Autodesk Inventor part; units mm, degrees
ref_plane "IP1_XY" through (0, 0, 0) normal (1, 0, 0) x (0, 0, -1)
ref_plane "IP1_YZ" through (0, 0, 0) normal (0, 0, -1) x (0, 1, 0)
ref_plane "IP1_ZX" through (0, 0, 0) normal (0, 1, 0) x (1, 0, 0)
sketch "Skizze_5" plane through (0, 0, 0) normal (0, 0, 1) x (1, 0, 0)
  line L0 (8, 0) -> (0, 0)
  line L1 (0, 0) -> (0, 3.75)
  line L2 (0, 3.75) -> (0.45, 3.75)
  line L3 (0.45, 3.75) -> (2.2, 2)
  line L4 (2.2, 2) -> (7.5705, 2)
  line L5 (7.5705, 2) -> (8, 1.5705)
  line L6 (8, 1.5705) -> (8, 0)
  line L7 (8, 0) -> (0, 0)
revolve "Revolution1" add sketch "Skizze_5" angle 360 about axis through (8, 0, 0) along (1, 0, 0)
thread "Thread1"
sketch "Sketch_1" plane through (0, 0, 0) normal (0, 0, 1) x (1, 0, 0)
  line L0 (1.66, 0) -> (0, 0)
  line L1 (0, 0) -> (0, 1.975)
  line L2 (0, 1.975) -> (1.66, 1.975)
  line L3 (1.66, 1.975) -> (1.66, 0)
  line L4 (1.66, 0) -> (0, 0)
revolve "Revolution2" cut sketch "Sketch_1" angle 360 about axis through (1.66, 0, 0) along (1, 0, 0)
sketch "Sketch_2" plane through (0, 0, 0) normal (0, 0, 1) x (1, 0, 0)
  line L0 (2.8003, 0) -> (1.66, 0)
  line L1 (1.66, 0) -> (1.66, 1.975)
  line L2 (1.66, 1.975) -> (2.8003, 0)
  line L3 (2.8003, 0) -> (1.66, 0)
revolve "Revolution3" cut sketch "Sketch_2" angle 360 about axis through (2.8003, 0, 0) along (1, 0, 0)
sketch "Sketch_3" plane through (0, 0, 0) normal (1, 0, 0) x (0, 1, 0)
  circle A0 centre (0, 0) radius 2.37
  arc A1 (-0.5027, 1.6394) -> (-1.1684, 1.2551) centre (-0.79, 1.3683) ccw
  arc A2 (-1.6711, 0.3843) -> (-1.1684, 1.2551) centre (-1.8307, 1.0569) ccw
  arc A3 (-1.6711, 0.3843) -> (-1.6711, -0.3843) centre (-1.58, 0) ccw
  arc A4 (-1.1684, -1.2551) -> (-1.6711, -0.3843) centre (-1.8307, -1.0569) ccw
  arc A5 (-1.1684, -1.2551) -> (-0.5027, -1.6394) centre (-0.79, -1.3683) ccw
  arc A6 (0.5027, -1.6394) -> (-0.5027, -1.6394) centre (0, -2.1139) ccw
  arc A7 (0.5027, -1.6394) -> (1.1684, -1.2551) centre (0.79, -1.3683) ccw
  arc A8 (1.6711, -0.3843) -> (1.1684, -1.2551) centre (1.8307, -1.0569) ccw
  arc A9 (1.6711, -0.3843) -> (1.6711, 0.3843) centre (1.58, 0) ccw
  arc A10 (1.1684, 1.2551) -> (1.6711, 0.3843) centre (1.8307, 1.0569) ccw
  arc A11 (1.1684, 1.2551) -> (0.5027, 1.6394) centre (0.79, 1.3683) ccw
  arc A12 (-0.5027, 1.6394) -> (0.5027, 1.6394) centre (0, 2.1139) ccw
extrude "Extrusion1" add sketch "Sketch_3" along normal blind 1.66
sketch "Sketch_4" plane through (0, 0, 0) normal (0, 0, 1) x (1, 0, 0)
  line L0 (1.1403, 0) -> (-1.66, 0)
  line L1 (-1.66, 0) -> (-1.66, 1.975)
  line L2 (-1.66, 1.975) -> (0, 1.975)
  line L3 (0, 1.975) -> (1.1403, 0)
  line L4 (1.1403, 0) -> (-1.66, 0)
revolve "Revolution4" cut sketch "Sketch_4" angle 360 about axis through (1.1403, 0, 0) along (1, 0, 0)
ref_plane "IP1_XY" through (0, 0, 0) normal (1, 0, 0) x (0, 0, -1)
ref_plane "IP1_YZ" through (0, 0, 0) normal (0, 0, -1) x (0, 1, 0)
ref_plane "IP1_ZX" through (0, 0, 0) normal (0, 1, 0) x (1, 0, 0)
ref_plane "IP2_XY" through (2.2, 0, 0) normal (1, 0, 0) x (0, 0, -1)
ref_plane "IP2_YZ" through (2.2, 0, 0) normal (0, 0, -1) x (0, 1, 0)
ref_plane "IP2_ZX" through (2.2, 0, 0) normal (0, 1, 0) x (1, 0, 0)
ref_plane "IP3_XY" through (8, 0, 0) normal (1, 0, 0) x (0, 0, -1)
ref_plane "IP3_YZ" through (8, 0, 0) normal (0, 0, -1) x (0, 1, 0)
ref_plane "IP3_ZX" through (8, 0, 0) normal (0, 1, 0) x (1, 0, 0)
properties part number "Senkschraube DIN ≈965 M4x8 51305.040.008(High)"
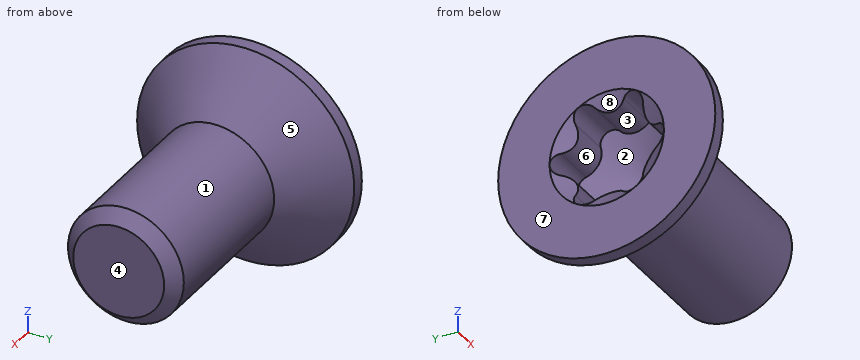
Here's how the part is built. I have some questions about the finished solid (model axes, mm). Face numbers are marked on the shaded views. A direction names the side the tool comes from. Round coordinates to 2 decimals unless told otherwise and drop trailing zeros. Order: outer loops, then holes, each group sorted by start corner. A loop starts at its lowest first (then second) coordinate and runs counter-clockwise, first axis right, second up. Notation, with made-up numbers: M 34.25,33 L 57.25,33 A34 cw 57.25,63 Z; hole C 56,88.25 d7. An arc over 180 degrees is marked long. One line per question, with ' | ' between items.
1) Imagine slicing it at A-A, the plane x = 6.5. Write out the boundary of the cut face in (y, z), plus the area to 3 significant figures.
Checked values:
outline: C 0,0 d4 | area: 12.6 mm²
2) We'd pull the mould along Y, two halves only. Please class the marked faces 5, 6, 7 and 8: released by +Y, released by -Y, zero draft, split by the parting line, or undercut.
Checked values:
face 5: split by the parting line | face 6: undercut | face 7: zero draft | face 8: undercut
3) I'm going to push flat-ended pins straight in: pin 1 Ø2 at (x, z) = (6.5, 1.5) entering from +Y; pin 2 Ø1.5 at (x, z) = (4, -2) entering from +Y; pin 3 Ø1 at (x, z) = (6.5, 0) entering from +Y; pin 4 Ø2 at (y, z) = (-0.5, -2) entering from +X. Where does each tip first touch, or does it pass through?
Checked values:
pin 1: stops at y = 1.94 | pin 2: stops at y = 1.56 | pin 3: stops at y = 2 | pin 4: stops at x = 8
4) I need wall thicknesses on line 1 (Z direction, x = 6, y = 0); line 2 (Z direction, x = 2, y = -0.75); line 3 (X direction, y = 2.75, z = -1.5). Which ranges of each line are inside material? Lowest first, please.
Checked values:
line 1: z = -2 to 2 | line 2: z = -2.07 to -1.17, 1.17 to 2.07 | line 3: x = 0 to 1.07
5) On a 3-axis mill with a long thin cutter (end or side, diameter ignored), from which of +Z, -Z, +X, -X, +Y, -Y can I reach the whole of each face in a straight line? I mean the marked faces 1, 2, 3 and 4. Say none if no direction works.
Checked values:
face 1: +X | face 2: none | face 3: -X | face 4: +Z, -Z, +X, +Y, -Y
